Here's the drawing with two shaded views (mm, measured from the low corner). I have some questions. A direction names the side the tool comes from. Coordinates: 2 decimals unless noted, no trailing zeros. Order: outer loops, then holes, each group sorted by start corner. A loop starts at its lowest first (then second) coordinate and runs counter-clockwise, first axis right, second up. Notation, with made-up numbers: (42, 60) - (71, 60) arc R30 cw to (71, 83) - close; hole circle Ø10 at (57.25, -37). An arc over 180 degrees is marked (long way). Answer as a JSON object with one key per item and string values. Group by question number.
(1) Please list where these lines run through material, in increasing order: probe 1 along X at (y, z) = (7.75, 2); probe 2 along Y at (x, z) = (14.5, 3.75); probe 3 along Y at (x, z) = (9.25, 1.5).
(2) Which directions (+Z, -Z, +X, -X, +Y, -Y) give clear straight access to the entire face, cutting with the end or side of a thin tool? Please do the marked faces 5, 6 and 7.
(3) We'd pull the mould along Y, two halves only. Please class the marked faces 1, 2, 3 and 4: pulls with the +Y half, pulls with the -Y half, needs draft (parallel to the pull), parting line crosses it, or undercut.
(4) Imagine slicing it at B-B, the plane x = 14.5. Write out the boundary of the cut face in (y, z).
(5) Imagine slicing it at A-A, the plane y = 7.5. Write out the boundary of the cut face in (x, z), and give its area (3 significant figures).
(6) Imagine slicing it at D-D, the plane z = 1.5. Write out the boundary of the cut face in (x, y), and give its area (3 significant figures).
(7) Imagine slicing it at C-C, the plane y = 5. Write out the boundary of the cut face in (x, z), and give its area (3 significant figures).
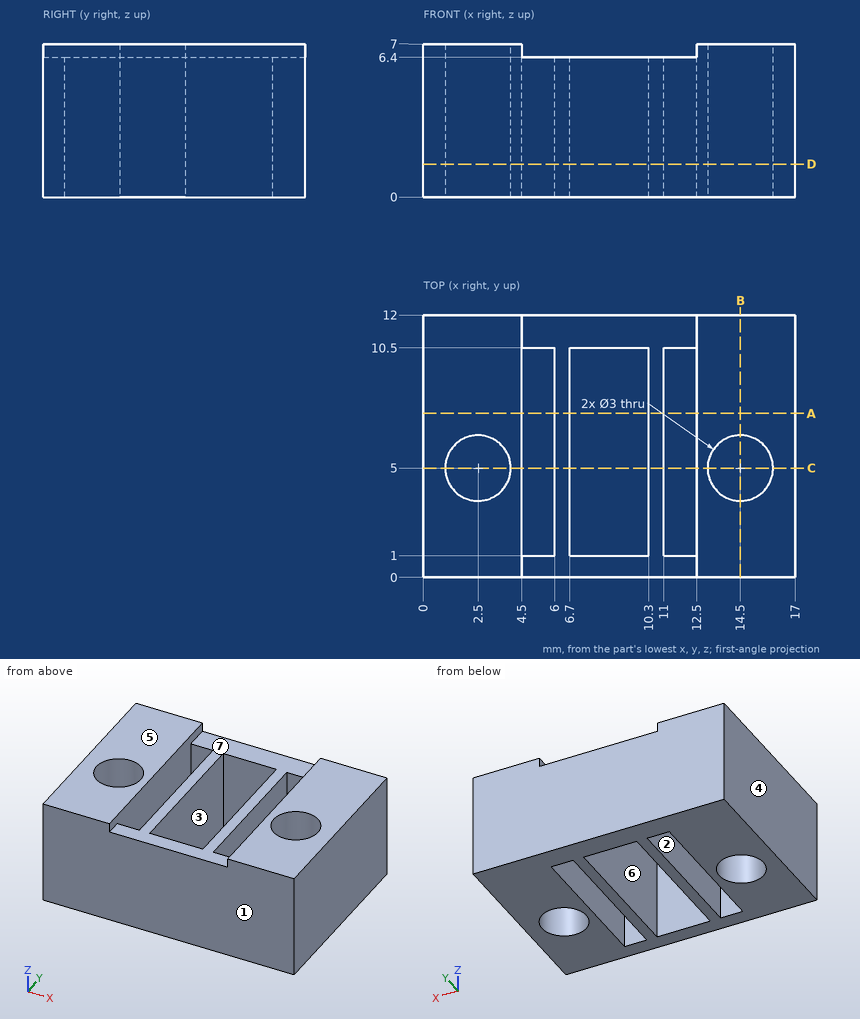
Result set:
{
 "1": {"probe 1": "x = 0 to 4.5, 6 to 6.7, 10.3 to 11, 12.5 to 17", "probe 2": "y = 0 to 3.5, 6.5 to 12", "probe 3": "y = 0 to 1, 10.5 to 12"},
 "2": {"face 5": "+Z, +X, -X, +Y, -Y", "face 6": "+Z, -Z", "face 7": "+Z, +Y, -Y"},
 "3": {"face 1": "pulls with the -Y half", "face 2": "undercut", "face 3": "undercut", "face 4": "needs draft"},
 "4": {"outline": "(0, 0) - (3.5, 0) - (3.5, 7) - (0, 7) - close; (6.5, 0) - (12, 0) - (12, 7) - (6.5, 7) - close"},
 "5": {"outline": "(0, 0) - (4.5, 0) - (4.5, 7) - (0, 7) - close; (6, 0) - (6.7, 0) - (6.7, 6.4) - (6, 6.4) - close; (10.3, 0) - (11, 0) - (11, 6.4) - (10.3, 6.4) - close; (12.5, 0) - (17, 0) - (17, 7) - (12.5, 7) - close", "area": "72.0 mm^2"},
 "6": {"outline": "(0, 0) - (17, 0) - (17, 12) - (0, 12) - close; hole circle Ø3 at (2.5, 5); hole (4.5, 1) - (6, 1) - (6, 10.5) - (4.5, 10.5) - close; hole (6.7, 1) - (10.3, 1) - (10.3, 10.5) - (6.7, 10.5) - close; hole (11, 1) - (12.5, 1) - (12.5, 10.5) - (11, 10.5) - close; hole circle Ø3 at (14.5, 5)", "area": "127 mm^2"},
 "7": {"outline": "(0, 0) - (1, 0) - (1, 7) - (0, 7) - close; (4, 0) - (4.5, 0) - (4.5, 7) - (4, 7) - close; (6, 0) - (6.7, 0) - (6.7, 6.4) - (6, 6.4) - close; (10.3, 0) - (11, 0) - (11, 6.4) - (10.3, 6.4) - close; (12.5, 0) - (13, 0) - (13, 7) - (12.5, 7) - close; (16, 0) - (17, 0) - (17, 7) - (16, 7) - close", "area": "30.0 mm^2"}
}
